Design review of the part built by this model. Coordinates are the model's own, in mm. Face numbers are marked on the shaded views. Coordinates: 2 decimals unless noted, no trailing zeros. Write each loop counter-clockwise with the first axis right and the second up, starting at its lowest first coordinate (ties: lowest second). Pieces come first, ordered by that corner, then holes. Notation, with made-up numbers: (32.25, 9.25) - (39.25, 9.25) arc R27 cw to (39.25, 29.25) - close; hole circle Ø8 at (-19, 29.5). An arc over 180 degrees is marked (long way). One line per item, written item: value.
from build123d import *

# Parameters (mm, degrees)
F1_DEPTH = 39
F2_R     = 4
F3_DEPTH = 3.6
F3_TAPER = 38


with BuildPart() as f1:
    # F0 (on Front) → F1 (new body)
    with BuildSketch(Plane.XZ):
        Polygon((7.6, 1.8), (-10.4, 1.8), (-10.4, 0), (-13.2, 0), (-13.2, -1.8), (10.4, -1.8), (10.4, 0), (7.6, 0), align=None)
    extrude(amount=-F1_DEPTH)

    # F2 (on face) → F3 (cut, through all)
    with BuildSketch(Plane(origin=(0, 0, -1.8), x_dir=(1, 0, 0), z_dir=(0, 0, -1))):
        with Locations((-1.4, -31)):
            Circle(F2_R)
        with Locations((-1.4, -19.5)):
            Circle(F2_R)
        with Locations((-1.4, -8)):
            Circle(F2_R)
    extrude(amount=-F3_DEPTH, taper=F3_TAPER, mode=Mode.SUBTRACT)


solid = f1.part
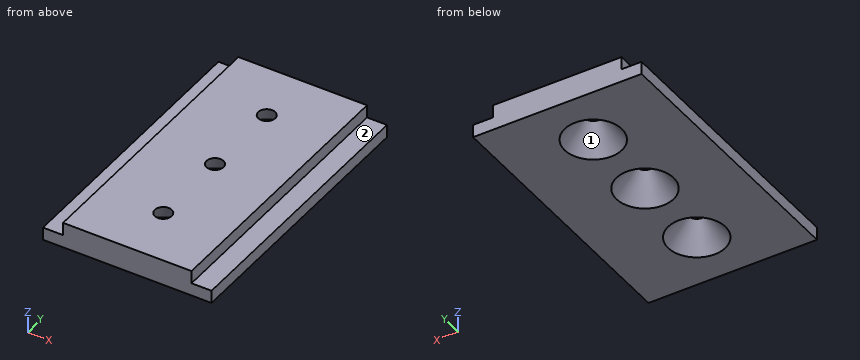
1. Consider section A-A, the plane y = 14. Write out the cut boundary in (x, z).
Answer block:
outline: (-13.2, -1.8) - (10.4, -1.8) - (10.4, 0) - (7.6, 0) - (7.6, 1.8) - (-10.4, 1.8) - (-10.4, 0) - (-13.2, 0) - close
2. Insertion check: pin 1 Ø0.8 at (x, y) = (-11.5, 17) entering from +Z; pin 2 Ø2 at (y, z) = (12.5, 0.5) entering from +X; pin 3 Ø0.5 at (y, z) = (20, 1.5) entering from -X. Each pin has a flat end and moves straight along its axis. Give the tip position at first contact, or say it passes through.
Answer block:
pin 1: stops at z = 0
pin 2: stops at x = 10.4
pin 3: stops at x = -10.4
3. Consider section C-C, the plane z = -0.45. Write out the cut boundary in (x, y).
Answer block:
outline: (-13.2, 0) - (10.4, 0) - (10.4, 39) - (-13.2, 39) - close; hole circle Ø5.89 at (-1.4, 8); hole circle Ø5.89 at (-1.4, 19.5); hole circle Ø5.89 at (-1.4, 31)
4. Mouldability with a two-part tool opening along X and no side actions: class the marked faces 1 and 2 as released by +X, released by -X, zero draft, split by the parting line, or undercut.
Answer block:
face 1: undercut
face 2: zero draft
5. Wall thickness on line 1 along Y through (x, z) = (-2.5, -1.4); line 2 along X through (y, z) = (8, 1.25); line 3 along X through (y, z) = (20, 0.15): over which ranges is each line inside the solid? List them lowest first.
Answer block:
line 1: y = 0 to 4.48, 11.52 to 15.98, 23.02 to 27.48, 34.52 to 39
line 2: x = -10.4 to -3.02, 0.22 to 7.6
line 3: x = -10.4 to -3.83, 1.03 to 7.6
6. Consider section B-B, the plane x = -1.4. Write out the cut boundary in (y, z).
Answer block:
outline: (0, -1.8) - (4, -1.8) - (6.81, 1.8) - (0, 1.8) - close; (9.19, 1.8) - (12, -1.8) - (15.5, -1.8) - (18.31, 1.8) - close; (20.69, 1.8) - (23.5, -1.8) - (27, -1.8) - (29.81, 1.8) - close; (32.19, 1.8) - (35, -1.8) - (39, -1.8) - (39, 1.8) - close
